```python
from build123d import *

# Parameters (mm, degrees)
ESQUISSE1_R             = 4.1
BOSS_EXTRU_1_DEPTH      = 5
ESQUISSE2_R             = 10.1
ENL_V_MAT_EXTRU_1_DEPTH = 2.5
BOSS_EXTRU_2_START      = 8.25
BOSS_EXTRU_2_DEPTH      = 8.25
ENL_V_MAT_EXTRU_2_DEPTH = 58.586020219
CHANFREIN1_START        = -2.5
CHANFREIN1_DEPTH        = 5


with BuildPart() as part:
    # Esquisse1 → Boss.-Extru.1 (new, symmetric)
    with BuildSketch(Plane(origin=(0, 0, 0), x_dir=(0, 1, 0), z_dir=(0, 0, 1))):
        with BuildLine():
            ThreePointArc((-8.760260026, 2.463299468), (0, -9.1), (8.760260026, 2.463299468))
            ThreePointArc((8.760260026, 2.463299468), (4.584088783, 25.765676228), (4.968111267, 49.4362))
            ThreePointArc((4.968111267, 49.4362), (0, 55), (-4.968111267, 49.4362))
            ThreePointArc((-4.968111267, 49.4362), (-4.584088783, 25.765676228), (-8.760260026, 2.463299468))
        make_face()
        with Locations(Location((0, 0, 0), (0, 0, 270))):
            Circle(ESQUISSE1_R, mode=Mode.SUBTRACT)
    extrude(amount=BOSS_EXTRU_1_DEPTH, both=True)

    # Esquisse2 → Enlèv. mat.-Extru.1 (cut, symmetric)
    with BuildSketch(Plane(origin=(0, 0, 0), x_dir=(0, 1, 0), z_dir=(0, 0, 1))):
        Circle(ESQUISSE2_R)
    extrude(amount=ENL_V_MAT_EXTRU_1_DEPTH, both=True, mode=Mode.SUBTRACT)

    # Esquisse3 → Boss.-Extru.2 (add)
    with BuildSketch(Plane.XY.offset(5).offset(BOSS_EXTRU_2_START)):
        with BuildLine():
            Line((-29, 1.651149925), (-29, -4.366011007))
            ThreePointArc((-29, -4.366011007), (-24.994289146, -4.648817083), (-21, -5.062765073))
            Line((-21, -5.062765073), (-21, 1.651149925))
            Line((-21, 1.651149925), (-29, 1.651149925))
        make_face()
    extrude(amount=-BOSS_EXTRU_2_DEPTH)

    # Esquisse4 → Enlèv. mat.-Extru.2 (cut, through all)
    with BuildSketch(Plane(origin=(0, 1.651149925, 0), x_dir=(-1, 0, 0), z_dir=(0, 1, 0))):
        Polygon((22.500084499, 8.25), (25, 10.25), (27.499915501, 8.25), (25, 6.25), align=None)
    extrude(amount=-ENL_V_MAT_EXTRU_2_DEPTH, mode=Mode.SUBTRACT)

    # Chanfrein1: read off the stored shape, not the designer's step
    # Chanfrein1 outline → Chanfrein1 (cut)
    with BuildSketch(Plane.XY.offset(CHANFREIN1_START)):
        with BuildLine():
            ThreePointArc((-6.552176852, 7.68628509), (-7.902187824, 7.364580252), (-9.255756722, 7.058190199))
            Line((-9.255756722, 7.058190199), (-9.253811974, 4.046846174))
            ThreePointArc((-9.253811974, 4.046846174), (-8.109790355, 6.020074784), (-6.552176852, 7.68628509))
        make_face()
    extrude(amount=CHANFREIN1_DEPTH, mode=Mode.SUBTRACT)


solid = part.part
```
Part model, mm, in its own coordinate system. A direction names the side the tool comes from. Round coordinates to 2 decimals unless told otherwise and drop trailing zeros. Write each loop counter-clockwise with the first axis right and the second up, starting at its lowest first coordinate (ties: lowest second). Pieces come first, ordered by that corner, then holes. Notation, with made-up numbers: M -18,75 L -11,75 A31 cw -11,106 Z; hole C 86.25,-9 d9. An arc over 180 degrees is marked long. Answer as CSV lines item,"result". Start each with the question number.
1) Band-saw the part on A-A (y = 0). List the corners of the cut face in (x, z), then the cut area to 3 significant figures.
2) Band-saw the part on B-B (x = 0). List the corners of the cut face in (y, z), then the cut area to 3 significant figures.
3) Mould opens along Z. For faces 1 (the face through (-23, 0, -5)), 2 (the face through (-23.733, -1.575, 9.236)), 3 (the face through (-26, 1.651, 10)), 4 (the face through (-23.768, -1.575, 7.236)) say: +Z half, -Z half, draft (parallel to the pull), parting line (faces both ways), or undercut.
4) Drop flat-ended pins along their axis: pin 1 (8 mm diameter, centred on y = 2, z = 10.5, fed in from -X); pin 2 (2 mm diameter, centred on x = -12.5, z = 6.5, fed in from +Y); pin 3 (10 mm diameter, centred on x = 0, y = -7, fed in from +Z); pin 4 (9 mm diameter, centred on x = -23.5, z = 8.5, fed in from +Y). Give the stop position or say it passes through.
5) Which spindle directions (+Z, -Z, +X, -X, +Y, -Y) get a long thin tool onto all of the face, cutting with end or side? Do faces 5 (the face through (-25, -2, 13.25)), 6 (the face through (-29, -1, 9)), 7 (the face through (-9.86, -2.18, 0.04)), 8 (the face through (-21, -2, 9)), 9 (the face through (-0.534, 4.065, -3.768)). Say none if no direction does.
6) Band-saw the part on C-C (z = 7). List the corners of the cut face in (x, y).
7) Drill centre lines: L1, parallel to Y at x = 0, z = 4.5; L2, parallel to X at y = 0, z = -3.6; L3, parallel to Z at x = -1.5, y = 6. Where is each one in solid material? Low to high.
8) Band-saw the part on D-D (x = -26.5). List the corners of the cut face in (y, z).
Worked out:
1,outline,"M -55,-5 L -4.1,-5 L -4.1,-2.5 L -10.1,-2.5 L -10.1,2.5 L -4.1,2.5 L -4.1,5 L -21,5 L -21,13.25 L -29,13.25 L -29,5 L -55,5 Z; M 4.1,-5 L 9.1,-5 L 9.1,-2.5 L 4.1,-2.5 Z; M 4.1,2.5 L 9.1,2.5 L 9.1,5 L 4.1,5 Z; hole M -27.5,8.25 L -25,6.25 L -22.5,8.25 L -25,10.25 Z"
1,area,"560 mm²"
2,outline,"M -9.1,-5 L -4.1,-5 L -4.1,-2.5 L -9.1,-2.5 Z; M -9.1,2.5 L -4.1,2.5 L -4.1,5 L -9.1,5 Z; M 4.1,-5 L 9.1,-5 L 9.1,-2.5 L 4.1,-2.5 Z; M 4.1,2.5 L 9.1,2.5 L 9.1,5 L 4.1,5 Z"
2,area,"50.0 mm²"
3,face 1,"-Z half"
3,face 2,"undercut"
3,face 3,"draft"
3,face 4,"undercut"
4,pin 1,"x = -29"
4,pin 2,"through"
4,pin 3,"z = 5"
4,pin 4,"y = 5.1"
5,face 5,"+Z, +X, -X, +Y, -Y"
5,face 6,"+Z, -X, +Y, -Y"
5,face 7,"+X"
5,face 8,"+Z, +X, +Y, -Y"
5,face 9,"+Z, -Z"
6,outline,"M -29,-4.37 A122.5 cw -25.94,-4.57 L -25.94,1.65 L -29,1.65 Z; M -24.06,-4.73 A122.5 cw -21,-5.06 L -21,1.65 L -24.06,1.65 Z"
7,L1,"-9.1 to -4.1, 4.1 to 9.1"
7,L2,"-55 to -4.1, 4.1 to 9.1"
7,L3,"-5 to -2.5, 2.5 to 5"
8,outline,"M -4.53,-5 L 4.53,-5 L 4.53,5 L 1.65,5 L 1.65,7.45 L -4.53,7.45 Z; M -4.53,9.05 L 1.65,9.05 L 1.65,13.25 L -4.53,13.25 Z"
